Verification items for the finished model (mm, model axes). A direction names the side the tool comes from. Round coordinates to 2 decimals unless told otherwise and drop trailing zeros. Loops run counter-clockwise (first coordinate to the right, second up) from the corner with the lowest first, then second, coordinate; pieces in that order, holes last. Notation, with made-up numbers: M 89,31.5 L 135,31.5 A23 cw 135,55.5 Z; hole C 16,-37 d5. An arc over 180 degrees is marked long. Answer as CSV lines item,"result".
```python
from build123d import *

# Parameters (mm, degrees)
F1_DEPTH = 35
F2_W     = 40
F2_H     = 40
F3_DEPTH = 20
F5_DEPTH = 40
F4_R     = 9.5
F6_DEPTH = 40


with BuildPart() as f1:
    # F0 (on Front) → F1 (new body)
    with BuildSketch(Plane.XZ):
        with BuildLine():
            Line((5, 20), (5, 0))
            Line((5, 0), (20, 0))
            Line((20, 0), (20, 80))
            Line((20, 80), (-20, 80))
            Line((-20, 80), (-20, 0))
            Line((-20, 0), (-5, 0))
            Line((-5, 0), (-5, 20))
            ThreePointArc((-5, 20), (0, 25), (5, 20))
        make_face()
    extrude(amount=F1_DEPTH)

    # F2 (on face) → F3 (join)
    with BuildSketch(Plane.XZ.offset(35)):
        with Locations((0, 60)):
            Rectangle(F2_W, F2_H)
    extrude(amount=F3_DEPTH)

    # F4 (on face) → F5 (join)
    with BuildSketch(Plane.YZ.offset(20)):
        with BuildLine():
            Line((-65, 70), (-65, 50))
            ThreePointArc((-65, 50), (-62.071068, 42.928932), (-55, 40))
            Line((-55, 40), (-55, 80))
            ThreePointArc((-55, 80), (-62.071068, 77.071068), (-65, 70))
        make_face()
    extrude(amount=-F5_DEPTH)

    # F4 (on face) → F6 (cut)
    with BuildSketch(Plane.YZ.offset(20)):
        with Locations((-45, 60)):
            Circle(F4_R)
    extrude(amount=-F6_DEPTH, mode=Mode.SUBTRACT)


solid = f1.part
```
1) Go/stop test with flat-tipped pins: pin 1 (16 mm diameter, centred on x = 3, y = -47.5, fed in from -Z); pin 2 (12 mm diameter, centred on x = -10, z = 15.5, fed in from -Y). Record where each tip stops, or that it passes through.
Here are the results:
pin 1,"stops at z = 40"
pin 2,"stops at y = -35"
2) Section check C-C (x = 6). Record the cut outline in (y, z).
Here are the results:
outline,"M -65,50 A10 ccw -55,40 L -35,40 L -35,0 L 0,0 L 0,80 L -55,80 A10 ccw -65,70 Z; hole C -45,60 d19"
3) Section check D-D (y = -29). Record the cut outline in (x, z), plus the area to 3 significant figures.
Here are the results:
outline,"M -20,0 L -5,0 L -5,20 A5 cw 5,20 L 5,0 L 20,0 L 20,80 L -20,80 Z"
area,"2,960 mm^2"
4) Set-up check for faces 4 (the flat face through (-5, -17, 10)), 5 (the flat face through (0, -45, 40)), 6 (the flat face through (0, 0, 41)): record each of +Z, -Z, +X, -X, +Y, -Y from which the full face is reachable in a straight line by a thin tool's end or side.
Here are the results:
face 4,"-Z, +Y, -Y"
face 5,"-Z, +X, -X, -Y"
face 6,"+Z, -Z, +X, -X, +Y"
5) Material ranges on probe 1 along Z at (x, y) = (9, -45); probe 2 along X at (y, z) = (-8.5, 14); probe 3 along Y at (x, z) = (5, 39.5), recorded low to high.
Here are the results:
probe 1,"z = 40 to 50.5, 69.5 to 80"
probe 2,"x = -20 to -5, 5 to 20"
probe 3,"y = -35 to 0"
6) Section check A-A (z = 60). Record the cut outline in (x, y), plus the area to 3 significant figures.
Here are the results:
outline,"M -20,-65 L 20,-65 L 20,-54.5 L -20,-54.5 Z; M -20,-35.5 L 20,-35.5 L 20,0 L -20,0 Z"
area,"1,840 mm^2"
7) Section check B-B (y = -45). Record the cut outline in (x, z).
Here are the results:
outline,"M -20,40 L 20,40 L 20,50.5 L -20,50.5 Z; M -20,69.5 L 20,69.5 L 20,80 L -20,80 Z"
8) Draft check along X on faces 1 (the flat face through (5, -17, 10)), 2 (the flat face through (0, -65, 60)), 3 (the flat face through (-20, -26, 49)). Enter one of: +X half, -X half, draft (parallel to the pull), parting line (faces both ways), or undercut.
Here are the results:
face 1,"undercut"
face 2,"draft"
face 3,"-X half"
